Work out the finished part from the listing and answer in its coordinate system (mm). A direction names the side the tool comes from. Round coordinates to 2 decimals unless told otherwise and drop trailing zeros. Loops run counter-clockwise (first coordinate to the right, second up) from the corner with the lowest first, then second, coordinate; pieces in that order, holes last. Notation, with made-up numbers: (57.25, 74.25) - (68.25, 74.25) arc R25 ccw to (68.25, 112.25) - close; hole circle Ø8 at (-5.5, 64.5). An arc over 180 degrees is marked (long way). Answer as CSV lines item,"result". Start each with the question number.
Q1. Each of these flat-tipped pins is pushed along its axis until it touches: pin 1 Ø2 at (y, z) = (1, 0) entering from -X; pin 2 Ø0.7 at (x, z) = (-42, 54) entering from +Y; pin 3 Ø1.6 at (y, z) = (0.5, 2) entering from +X; pin 4 Ø1.5 at (y, z) = (4, 34.5) entering from -X. Where does it stop, or does it pass through?
Q2. Section B-B on x = -6 is taken. Write down the section's boundary in (y, z).
Q3. For faces 1 (the face through (-37.12, 1.01, 62.49)), 2 (the face through (1.1, 1, 54.1)), 3 (the face through (-24.46, 3.54, 2.18)), determine the directions among +Z, -Z, +X, -X, +Y, -Y from which every point of the face is accessible in a straight line to the end or side of a thin tool.
Q4. Straight lines are drawn through the part: L1, parallel to Z at x = 63.9, y = 1.55; L2, parallel to X at y = 0.55, z = 54; L3, parallel to X at y = 1.1, z = 54. For each, find the intervals that lie inside material, in ascending order. Write a range as [from, to].
Q5. The mould has two halves that part along Z. Classify faces 4 (the face through (-101.9, 1, 61)), 5 (the face through (3.19, 1.01, 62.56)), 6 (the face through (4, 2, 54)): +Z half, -Z half, draft (parallel to the pull), parting line (faces both ways), or undercut.
Q6. Section C-C on z = 39 is taken. Write down the section's boundary in (x, y).
Q7. Section A-A on y = 4.3 is taken. Write down the section's boundary in (x, z).
Autodesk Inventor part; units mm, degrees
ref_plane "YZ Plane" through (0, 0, 0) normal (1, 0, 0) x (0, 1, 0)
ref_plane "XZ Plane" through (0, 0, 0) normal (0, 1, 0) x (-1, 0, 0)
ref_plane "XY Plane" through (0, 0, 0) normal (0, 0, 1) x (1, 0, 0)
sketch "Sketch1" plane through (0, 0, 0) normal (0, 1, 0) x (-1, 0, 0)
  circle A0 centre (-13, 3.6355) radius 1.25
  circle A1 centre (47, 3.6355) radius 1.25
  circle A2 centre (-63.9, 60.95) radius 1.55
  circle A3 centre (-63.9, 60.95) radius 1.5
  circle A4 centre (97.9, 60.95) radius 1.55
  circle A5 centre (97.9, 60.95) radius 1.5
  arc A6 (47, -0.3645) -> (51, 3.6355) centre (47, 3.6355) ccw construction
  arc A7 (-17, 3.6395) -> (-13, -0.3645) centre (-13, 3.6355) ccw construction
  arc A8 (-63.9, 64.95) -> (-63.9, 56.95) centre (-63.9, 60.95) ccw
  arc A9 (97.9, 56.95) -> (97.9, 64.95) centre (97.9, 60.95) ccw
  line L0 (-13, -0.3645) -> (47, -0.3645) construction
  line L1 (-63.9, 64.95) -> (97.9, 64.95)
  line L2 (-17, 3.6395) -> (-17, 6.1391)
  line L3 (51, 3.6355) -> (51, 6.1391)
  arc A10 (51, 3.6355) -> (47, -0.3645) centre (47, 3.6355) ccw construction
  arc A11 (-13, -0.3645) -> (-17, 3.6395) centre (-13, 3.6355) ccw construction
  line L4 (-63.9, 56.95) -> (-61.722, 56.95)
  line L5 (97.9, 56.95) -> (95.722, 56.95)
  line L6 (92.7041, 55.5753) -> (51.9821, 8.7645)
  line L7 (-58.7041, 55.5753) -> (-17.9821, 8.7645)
  arc A12 (-58.7041, 55.5753) -> (-61.722, 56.95) centre (-61.722, 52.95) ccw
  arc A13 (95.722, 56.95) -> (92.7041, 55.5753) centre (95.722, 52.95) ccw
  arc A14 (51.9821, 8.7645) -> (51, 6.1391) centre (55, 6.1391) ccw
  arc A15 (-17, 6.1391) -> (-17.9821, 8.7645) centre (-21, 6.1391) ccw
  arc A16 (-63.9, 56.95) -> (-63.9, 64.95) centre (-63.9, 60.95) ccw construction
  arc A17 (97.9, 64.95) -> (97.9, 56.95) centre (97.9, 60.95) ccw construction
  line L8 (51, 3.6355) -> (51, -2.3645)
  line L9 (49, -4.3645) -> (-15, -4.3645)
  line L10 (-17, -2.3645) -> (-17, 3.6395)
  arc A18 (49, -4.3645) -> (51, -2.3645) centre (49, -2.3645) ccw
  arc A19 (-17, -2.3645) -> (-15, -4.3645) centre (-15, -2.3645) ccw
  line L11 (-13, 3.6355) -> (-13, 0.6355) construction
  line L12 (-14.25, 3.6355) -> (-14.25, 0.6355)
  line L13 (-11.75, 0.6355) -> (-11.75, 3.6355)
  arc A20 (-11.75, 3.6355) -> (-14.25, 3.6355) centre (-13, 3.6355) ccw
  arc A21 (-14.25, 0.6355) -> (-11.75, 0.6355) centre (-13, 0.6355) ccw
  line L14 (47, 3.6355) -> (47, 0.6355) construction
  line L15 (45.75, 3.6355) -> (45.75, 0.6355)
  line L16 (48.25, 0.6355) -> (48.25, 3.6355)
  arc A22 (48.25, 3.6355) -> (45.75, 3.6355) centre (47, 3.6355) ccw
  arc A23 (45.75, 0.6355) -> (48.25, 0.6355) centre (47, 0.6355) ccw
  point P0 (0, 0)
  point P1 (17, 90.5)
  point P2 (51, -4.3645)
  point P3 (-13, 2.1355)
  point P4 (47, 2.1355)
  point P5 (-11.75, 3.6355)
  dimension "d0" = 2.5
  dimension "d1" = 2.5
  dimension "d2" = 3
  dimension "d3" = 3
  dimension "d4" = 8
  dimension "d5" = 8
  dimension "d6" = 8
  dimension "d7" = 8
  dimension "d8" = 60
  dimension "d18" = 4
  dimension "d313" = 8
  dimension "d314" = 2
  dimension "d322" = 3
  dimension "d323" = 3
extrude "Extrusion1" add sketch "Sketch1" along normal blind 2 contours L1 A9 L5 A13 L6 A14 L3 L8 A18 L9 A19 L10 L2 A15 L7 A12 L4 A8
sketch "Sketch3" plane through (0, 2, 0) normal (0, 1, 0) x (1, 0, 0)
  circle A0 centre (13, -3.6355) radius 1.55 construction
  line L0 (13, -3.6355) -> (-2, 2) construction
  line L1 (-2, 2) -> (-2, 4) construction
  line L2 (-2, 2) -> (-2, 4) construction
  line L3 (-2, 4) -> (6, 6.8723) construction
  line L4 (9.8, 6.8723) -> (53.9673, -18.6277) construction
  line L5 (6, 6.8723) -> (9.8, 6.8723) construction
  line L6 (9.8, 6.8723) -> (53.9673, -18.6277) construction
  line L7 (57.4673, -24.6899) -> (57.0036, -33.6779) construction
  line L8 (53.9673, -18.6277) -> (57.4673, -24.6899) construction
  line L9 (57.4673, -24.6899) -> (57.0036, -33.6779) construction
  line L10 (75.376, -65.5) -> (80.5, -65.5) construction
  line L11 (57.0036, -33.6779) -> (75.376, -65.5) construction
  line L12 (75.376, -65.5) -> (6.5, -65.7) construction
  line L13 (6.5, -65.7) -> (6.2893, -65.5) construction
  line L14 (0.6, -60.1) -> (-9.5, -60.1)
  line L15 (-9.5, -60.1) -> (-11, -62.1)
  line L16 (-9.5, -60.1) -> (-11, -62.1)
  line L17 (-23, -62.1) -> (-11, -62.1)
  line L18 (-11, -62.1) -> (-23, -62.1)
  line L19 (-24.5, -60.1) -> (-23, -62.1)
  line L20 (-23, -62.1) -> (-24.5, -60.1)
  line L21 (-34.6, -60.1) -> (-24.5, -60.1)
  line L22 (-24.5, -60.1) -> (-34.6, -60.1)
  line L23 (-40.5, -71.9) -> (-40.5, -65.7) construction
  line L24 (-34.6, -60.1) -> (-39.7098, -64.95)
  line L25 (-114.5, -65.5) -> (-109.376, -65.5) construction
  line L26 (-40.5, -65.7) -> (-109.376, -65.5) construction
  line L27 (-109.376, -65.5) -> (-91.0036, -33.6779) construction
  line L28 (-87.9673, -18.6277) -> (-91.4673, -24.6899) construction
  line L29 (-91.0036, -33.6779) -> (-91.4673, -24.6899) construction
  line L30 (-91.4673, -24.6899) -> (-87.9673, -18.6277) construction
  line L31 (-40, 6.8723) -> (-43.8, 6.8723) construction
  line L32 (-87.9673, -18.6277) -> (-43.8, 6.8723) construction
  line L33 (-43.8, 6.8723) -> (-40, 6.8723) construction
  line L34 (-32, 4) -> (-40, 6.8723) construction
  line L35 (-40, 6.8723) -> (-32, 4) construction
  line L36 (-32, 4) -> (-32, 2) construction
  line L37 (-32, 2) -> (-2, 2) construction
  line L38 (-6.4, -15.5) -> (-2.8831, -15.5)
  line L39 (-2.8831, -15.5) -> (-6.4, -15.5)
  line L40 (-26.1, -17.5) -> (-7.9, -17.5)
  line L41 (-6.4, -15.5) -> (-7.9, -17.5)
  line L42 (-7.9, -17.5) -> (-26.1, -17.5)
  line L43 (-31.1169, -15.5) -> (-27.6, -15.5)
  line L44 (-26.1, -17.5) -> (-27.6, -15.5)
  line L45 (-35.1306, -20.7029) -> (-31.1169, -15.5)
  line L46 (-27.6, -15.5) -> (-31.1169, -15.5)
  line L47 (-31.1169, -15.5) -> (-35.1306, -20.7029)
  line L48 (-35.1306, -20.7029) -> (-27.0449, -36)
  line L49 (-22.7189, -36) -> (-27.0449, -36)
  line L50 (-27.0449, -36) -> (-22.7189, -36)
  line L51 (-20.9689, -37) -> (-22.7189, -36)
  line L52 (-22.7189, -36) -> (-20.9689, -37)
  line L53 (-13.0311, -37) -> (-20.9689, -37)
  line L54 (-20.9689, -37) -> (-13.0311, -37)
  line L55 (-11.2811, -36) -> (-13.0311, -37)
  line L56 (-13.0311, -37) -> (-11.2811, -36)
  line L57 (-6.9551, -36) -> (-11.2811, -36)
  line L58 (-11.2811, -36) -> (-6.9551, -36)
  line L59 (1.1306, -20.7029) -> (-6.9551, -36)
  line L60 (-6.9551, -36) -> (1.1306, -20.7029)
  line L61 (1.1306, -20.7029) -> (-2.8831, -15.5)
  arc A1 (11.75, -3.6355) -> (14.25, -3.6355) centre (13, -3.6355) ccw
  line L62 (-97.9, -64.95) -> (63.9, -64.95)
  line L63 (5.7098, -64.95) -> (-39.7098, -64.95)
  line L64 (5.7098, -64.95) -> (0.6, -60.1)
  point P0 (0, 0)
  point P1 (17, 90.5)
extrude "Extrusion3" cut sketch "Sketch3" against normal up to next contours L64 L62 L24 L21 L19 L17 L15 L14
sketch "Sketch16" plane through (0, 0, 0) normal (0, -1, 0) x (1, 0, 0)
  line L0 (-34.6, 60.1) -> (-39.7098, 64.95) construction
  line L1 (-34.6, 60.1) -> (-34.6, 54) construction
  line L2 (-34.6, 54) -> (-38.1, 54) construction
  circle A0 centre (-38.1, 54) radius 3
  circle A1 centre (4.1, 54) radius 3
  line L3 (0.6, 60.1) -> (-9.5, 60.1) construction
  point P0 (0, 0)
  dimension "d114" = 6.1
  dimension "d115" = 3.5
  dimension "d116" = 6
  dimension "d117" = 6
  dimension "d118" = 42.2
  dimension "d119" = 6.1
sketch "Sketch2" plane through (0, 2, 0) normal (0, 1, 0) x (1, 0, 0)
  arc A0 (11.75, -3.6355) -> (14.25, -3.6355) centre (13, -3.6355) ccw
  arc A1 (-48.25, -3.6355) -> (-45.75, -3.6355) centre (-47, -3.6355) ccw
  line L0 (13, 0.3645) -> (-47, 0.3645)
  circle A2 centre (-41.13, -53.4355) radius 4
  circle A3 centre (7.13, -54.7055) radius 4
  circle A4 centre (-25.89, -2.6355) radius 4
  point P0 (0, 0)
  point P1 (-28.5358, 0.3645)
  point P2 (-23.2442, 0.3645)
  dimension "d21" = 60
  dimension "d337" = 8
  dimension "d343" = 8
  dimension "d345" = 48.26
  dimension "d346" = 5.87
  dimension "d348" = 1.27
  dimension "d349" = 8
  dimension "d350" = 1
  dimension "d351" = 15.24
  dimension "d352" = 50.8
extrude "Extrusion2" add sketch "Sketch2" along normal blind 4
chamfer "Chamfer2" distance 3 distance2 4 3 edges at (-45.13, 2, 53.4355) (3.13, 2, 54.7055) (-28.5358, 2, 5.6355) measured on face at (28.9368, 2, 38.7976)
sketch "Sketch17" plane through (0, 2, 0) normal (0, 1, 0) x (1, 0, 0)
  arc A0 (11.75, -3.6355) -> (14.25, -3.6355) centre (13, -3.6355) ccw
  circle A1 centre (13, -3.6355) radius 2.5
  arc A2 (-48.25, -3.6355) -> (-45.75, -3.6355) centre (-47, -3.6355) ccw
  circle A3 centre (-47, -3.6355) radius 2.5
  line L0 (13, -3.6355) -> (13, 0) construction
  line L1 (15.5, -3.6355) -> (15.5, 0)
  line L2 (10.5, 0) -> (10.5, -3.6355)
  arc A4 (10.5, -3.6355) -> (15.5, -3.6355) centre (13, -3.6355) ccw
  arc A5 (15.5, 0) -> (10.5, 0) centre (13, 0) ccw
  line L3 (-47, -3.6355) -> (-47, 0) construction
  line L4 (-44.5038, -3.6355) -> (-44.5038, 0)
  line L5 (-49.4962, 0) -> (-49.4962, -3.6355)
  arc A6 (-49.4962, -3.6355) -> (-44.5038, -3.6355) centre (-47, -3.6355) ccw
  arc A7 (-44.5038, 0) -> (-49.4962, 0) centre (-47, 0) ccw
  point P0 (0, 0)
  point P1 (13, -1.8177)
  point P2 (-47, -1.8177)
  point P3 (-49.4962, -3.4982)
  point P4 (-44.5038, -3.4982)
  dimension "d125" = 5
  dimension "d126" = 5
extrude "Extrusion17" cut sketch "Sketch17" along normal through all
extrude "Extrusion18" cut sketch "Sketch16" against normal blind 2
sketch "Sketch22" plane through (-39.5, 6, 6.6355) normal (0, 1, 0) x (1, 0, 0)
  circle A0 centre (-1.63, -46.8) radius 4
  circle A1 centre (-1.63, -46.8) radius 1.5
  circle A2 centre (46.63, -48.07) radius 4
  circle A3 centre (46.63, -48.07) radius 1.5
  circle A4 centre (13.61, 4) radius 4
  circle A5 centre (13.61, 4) radius 1.5
  dimension "d339" = 3
  dimension "d347" = 3
  dimension "d353" = 3
extrude "Extrusion24" cut sketch "Sketch22" against normal blind 5 contours A1 | A3 | A5
properties part number "ArduSimple BasePlate FrontExit"
Findings:
1,pin 1,"stops at x = -51"
1,pin 2,"stops at y = 1"
1,pin 3,"stops at x = 17"
1,pin 4,"passes through"
2,outline,"(0, -4.36) - (2, -4.36) - (2, 60.1) - (0, 60.1) - close"
3,face 1,"+Z, +Y, -Y"
3,face 2,"-Y"
3,face 3,"+Y"
4,L1,"z = [56.95, 59.4], [62.5, 64.95]"
4,L2,"x = [-91.33, -41.1], [-35.1, 1.1], [7.1, 57.33]"
4,L3,"x = [-91.33, -42.52], [-35.1, 1.1], [8.45, 57.33]"
5,face 4,"parting line"
5,face 5,"+Z half"
5,face 6,"undercut"
6,outline,"(-78.28, 0) - (44.28, 0) - (44.28, 2) - (-78.28, 2) - close"
7,outline,"circle Ø10.55 at (-41.13, 53.44); circle Ø10.55 at (-25.89, 2.64); circle Ø10.55 at (7.13, 54.71); hole circle Ø3 at (-41.13, 53.44); hole circle Ø3 at (-25.89, 2.64); hole circle Ø3 at (7.13, 54.71)"
